from build123d import *

# Parameters (mm, degrees)
EXTRUDE_1_DEPTH     = 3
EXTRUDE_2_DEPTH     = 51
EXTRUDE_3_DEPTH     = 3
FILLET_1_R          = 3
CHAMFER_1_SIZE      = 0.5
SKETCH_4_W          = 5
SKETCH_4_H          = 40
CUT_EXTRUDE_1_DEPTH = 58.742047602
FILLET_2_R          = 2


with BuildPart() as part:
    # 草图1 → 凸台-拉伸1 (new body)
    with BuildSketch(Plane.XY):
        with BuildLine():
            Line((-4.299038106, 4.446152423), (-0.866025404, -1.5))
            Line((-0.866025404, -1.5), (6, -1.5))
            ThreePointArc((6, -1.5), (7.5, 0), (6, 1.5))
            Line((6, 1.5), (0.866025404, 1.5))
            Line((0.866025404, 1.5), (-1.700961894, 5.946152423))
            ThreePointArc((-1.700961894, 5.946152423), (-3.75, 6.495190528), (-4.299038106, 4.446152423))
        make_face()
    extrude(amount=EXTRUDE_1_DEPTH)

    # 草图2 → 凸台-拉伸2 (add)
    with BuildSketch(Plane.XY.offset(3)):
        with BuildLine():
            Line((-0.5, 6.696152423), (-3, 6.696152423))
            ThreePointArc((-3, 6.696152423), (-2.25, 6.495190528), (-1.700961894, 5.946152423))
            Line((-1.700961894, 5.946152423), (0.866025404, 1.5))
            Line((0.866025404, 1.5), (6, 1.5))
            ThreePointArc((6, 1.5), (7.060660172, 1.060660172), (7.5, 0))
            Line((7.5, 0), (7.5, 3))
            Line((7.5, 3), (1.633974596, 3))
            Line((1.633974596, 3), (-0.5, 6.696152423))
        make_face()
        with BuildLine():
            Line((-4.299038106, 4.446152423), (-0.866025404, -1.5))
            Line((-0.866025404, -1.5), (6, -1.5))
            ThreePointArc((6, -1.5), (7.060660172, -1.060660172), (7.5, 0))
            ThreePointArc((7.5, 0), (7.060660172, 1.060660172), (6, 1.5))
            Line((6, 1.5), (0.866025404, 1.5))
            Line((0.866025404, 1.5), (-1.700961894, 5.946152423))
            ThreePointArc((-1.700961894, 5.946152423), (-1.551111261, 5.58438099), (-1.5, 5.196152423))
            ThreePointArc((-1.5, 5.196152423), (-2.611771432, 3.747263683), (-4.299038106, 4.446152423))
        make_face()
        with BuildLine():
            ThreePointArc((-3, 6.696152423), (-4.299038106, 5.946152423), (-4.299038106, 4.446152423))
            ThreePointArc((-4.299038106, 4.446152423), (-2.611771432, 3.747263683), (-1.5, 5.196152423))
            ThreePointArc((-1.5, 5.196152423), (-1.551111261, 5.58438099), (-1.700961894, 5.946152423))
            ThreePointArc((-1.700961894, 5.946152423), (-2.25, 6.495190528), (-3, 6.696152423))
        make_face()
    extrude(amount=EXTRUDE_2_DEPTH)

    # 草图3 → 凸台-拉伸3 (add)
    with BuildSketch(Plane.XY.offset(54)):
        with BuildLine():
            Line((-4.299038106, 4.446152423), (-0.866025404, -1.5))
            Line((-0.866025404, -1.5), (6, -1.5))
            ThreePointArc((6, -1.5), (7.5, 0), (6, 1.5))
            Line((6, 1.5), (0.866025404, 1.5))
            Line((0.866025404, 1.5), (-1.700961894, 5.946152423))
            ThreePointArc((-1.700961894, 5.946152423), (-3.75, 6.495190528), (-4.299038106, 4.446152423))
        make_face()
    extrude(amount=EXTRUDE_3_DEPTH)

    # 圆角1
    fillet_1_edges = [part.edges().sort_by_distance(p)[0] for p in [
        (0.866025404, 1.5, 55.5),
        (7.5, 3, 28.5),
        (-0.5, 6.696152423, 28.5),
        (0.866025404, 1.5, 1.5),
        (-0.866025404, -1.5, 28.5),
    ]]
    fillet(fillet_1_edges, radius=FILLET_1_R - 0.0001)  # a hair under: the kernel refuses the full size

    # 倒角1
    chamfer_1_edges = [part.edges().sort_by_distance(p)[0] for p in [
        (7.5, 0, 57),
        (-3.75, 6.495190528, 57),
        (-3.015530023, 2.223051211, 57),
        (-0.850466513, 4.473051211, 57),
        (4.299009238, 1.5, 57),
        (-3.75, 6.495190528, 0),
        (-0.850466513, 4.473051211, 0),
        (4.299009238, 1.5, 0),
        (3.432983834, -1.5, 0),
        (3.432983834, -1.5, 57),
        (-3.015530023, 2.223051211, 0),
        (-0.633982331, -1.098089609, 0),
        (-0.633982331, -1.098089609, 57),
        (1.098068476, 1.901910391, 57),
        (1.098068476, 1.901910391, 0),
        (7.5, 0, 0),
    ]]
    chamfer(chamfer_1_edges, length=CHAMFER_1_SIZE)

    # 草图4 → 切除-拉伸1 (cut, through all)
    with BuildSketch(Plane(origin=(2.486112979, 4.528124648, 0), x_dir=(0.8765717103484919, -0.4812712713394804, 0), z_dir=(0.4812712713394804, 0.8765717103484919, 0))):
        with Locations((-0.011517908, -28.5)):
            Rectangle(SKETCH_4_W, SKETCH_4_H)
    extrude(amount=-CUT_EXTRUDE_1_DEPTH, mode=Mode.SUBTRACT)

    # 圆角2
    fillet_2_edges = [part.edges().sort_by_distance(p)[0] for p in [
        (-1.076934244, 3.257015136, 48.5),
        (3.250658802, 0.75, 48.5),
        (-1.076934244, 3.257015136, 8.5),
        (3.250658802, 0.75, 8.5),
    ]]
    fillet(fillet_2_edges, radius=FILLET_2_R)


solid = part.part
Geometry check sheet. Reference: the model listing, model coordinates, mm. A direction names the side the tool comes from. Give positions to 0.01 mm unless a question says otherwise; leave off trailing zeros. Answer as a JSON object with one key per item and string values. Group by question number.
Item 1: Mould release check, pull along X, two halves, no side actions. Record for faces 1 (the flat face through (-3.32, 2.75, 28.11)), 2 (the cylindrical face through (2.49, 0.61, 47.93)), 3 (the conical face through (7.14, -0.03, 0.14)): pulls with the +X half, pulls with the -X half, needs draft (parallel to the pull), parting line crosses it, or undercut.
Item 2: Gauge pin test, flat ends, axial feed: pin 1 (3 mm diameter, centred on x = 5, z = 2, fed in from +Y); pin 2 (4 mm diameter, centred on y = 3, z = 19.5, fed in from +X); pin 3 (3.5 mm diameter, centred on x = 1, y = 4.5, fed in from -Z). Record the tip position at first contact, or that the pin passes through.
Item 3: Access from +Z, -Z, +X, -X, +Y, -Y to the whole of each face (thin tool, end or side, straight path). Record for faces 4 (the cylindrical face through (6.64, 2.1, 28.86)), 5 (the flat face through (2.2, 2.6, 3)).
Item 4: Material ranges on L1, parallel to X at y = 0, z = 8; L2, parallel to Z at x = 7.25, y = 1; L3, parallel to Z at x = 0.75, y = -1, recorded low to high.
Findings below:
{
 "1": {"face 1": "pulls with the -X half", "face 2": "undercut", "face 3": "pulls with the +X half"},
 "2": {"pin 1": "y = 3", "pin 2": "x = 7.33", "pin 3": "z = 0.37"},
 "3": {"face 4": "+Z, -Z, +X, +Y", "face 5": "-Z, +X, +Y"},
 "4": {"L1": "-1.73 to 7.5", "L2": "3 to 54", "L3": "0 to 8.61, 48.39 to 57"}
}
